from build123d import *

# Parameters (mm, degrees)
F0_W     = 150
F0_H     = 110
F1_DEPTH = 50
F2_W     = 140
F2_H     = 100
F3_DEPTH = 45
F4_R     = 5
F6_DEPTH = 160


with BuildPart() as f1:
    # F0 (on Top) → F1 (new body)
    with BuildSketch(Plane.XY):
        Rectangle(F0_W, F0_H)
    extrude(amount=F1_DEPTH)

    # F2 (on face) → F3 (cut)
    with BuildSketch(Plane.XY.offset(50)):
        Rectangle(F2_W, F2_H)
    extrude(amount=-F3_DEPTH, mode=Mode.SUBTRACT)

    # F4
    f4_edges = [f1.edges().sort_by_distance(p)[0] for p in [
        (75, -55, 25),
        (75, 55, 25),
        (-75, 55, 25),
        (-75, -55, 25),
    ]]
    fillet(f4_edges, radius=F4_R)

    # F5 (on face) → F6 (cut)
    with BuildSketch(Plane.YZ.offset(75)):
        Polygon((10, 50), (-10, 50), (-15, 40), (15, 40), align=None)
    extrude(amount=-F6_DEPTH, mode=Mode.SUBTRACT)


solid = f1.part
The listing builds one solid part. Answer for the finished solid, in the listing's coordinates (mm). A direction names the side the tool comes from. Coordinates: 2 decimals unless noted, no trailing zeros. Write each loop counter-clockwise with the first axis right and the second up, starting at its lowest first coordinate (ties: lowest second). Pieces come first, ordered by that corner, then holes. Notation, with made-up numbers: (-40, 65) -> (19, 65) arc R26 ccw to (19, 91) -> close; hole circle Ø10 at (29.5, 3). An arc over 180 degrees is marked (long way). One line per question, with ' | ' between items.
1. Section B-B (y = 4) is taken. Determine the outline of the cut face in (x, z).
Verdict:
outline: (-75, 0) -> (75, 0) -> (75, 40) -> (70, 40) -> (70, 5) -> (-70, 5) -> (-70, 40) -> (-75, 40) -> close
2. Given pin 1 Ø1 at (x, y) = (-12, 35) entering from +Z; pin 2 Ø10 at (x, y) = (-46, 1) entering from -Z; pin 3 Ø1.5 at (x, y) = (-72.5, -3.5) entering from +Z, each flat-ended and moving along its own axis, determine where each tip first touches the part or whether it passes through.
Verdict:
pin 1: stops at z = 5 | pin 2: stops at z = 0 | pin 3: stops at z = 40
3. Which of the six approach directions +Z, -Z, +X, -X, +Y, -Y give full straight-line access (tool end or side, diameter ignored) to faces 1 (the flat face through (-1, 1, 0)), 2 (the flat face through (-72, 0, 40)), 3 (the flat face through (-70, -1, 28))?
Verdict:
face 1: -Z, +X, -X, +Y, -Y | face 2: +X, -X | face 3: +Z
4. Section A-A (z = 21) is taken. Determine the outline of the cut face in (x, y).
Verdict:
outline: (-75, -50) arc R5 ccw to (-70, -55) -> (70, -55) arc R5 ccw to (75, -50) -> (75, 50) arc R5 ccw to (70, 55) -> (-70, 55) arc R5 ccw to (-75, 50) -> close; hole (-70, -50) -> (70, -50) -> (70, 50) -> (-70, 50) -> close
5. Section C-C (x = -56.5) is taken. Determine the outline of the cut face in (y, z), and give its area (3 significant figures).
Verdict:
outline: (-55, 0) -> (55, 0) -> (55, 50) -> (50, 50) -> (50, 5) -> (-50, 5) -> (-50, 50) -> (-55, 50) -> close | area: 1,000 mm^2
6. Straight lines are drawn through the part: line 1 (X direction, y = -18, z = 39.5); line 2 (Y direction, x = 11, z = 27); line 3 (Z direction, x = -36, y = -3.5). For each, find the intervals that lie inside material, in ascending order.
Verdict:
line 1: x = -75 to -70, 70 to 75 | line 2: y = -55 to -50, 50 to 55 | line 3: z = 0 to 5
7. For a pull along Y with two mould halves and no side action, classify faces 4 (the flat face through (-1, 1, 5)), 5 (the flat face through (73, 0, 40)), 6 (the cylindrical face through (-74, 53, 25)), 7 (the flat face through (-75, -1, 25)) as released by +Y, released by -Y, zero draft, split by the parting line, or undercut.
Verdict:
face 4: undercut | face 5: undercut | face 6: released by +Y | face 7: zero draft
